from build123d import *

# Parameters (mm, degrees)
SKETCH2_W           = 100
SKETCH2_H           = 77
BOSS_EXTRUDE1_DEPTH = 18
SKETCH3_W           = 100
SKETCH3_H           = 24.402527788
CUT_EXTRUDE1_DEPTH  = 3.5


with BuildPart() as part:
    # Sketch2 → Boss-Extrude1 (new body)
    with BuildSketch(Plane.XY.offset(-10)):
        with Locations((45, 33.5)):
            Rectangle(SKETCH2_W, SKETCH2_H)
    extrude(amount=BOSS_EXTRUDE1_DEPTH)

    # Sketch3 → Cut-Extrude1 (cut)
    with BuildSketch(Plane.XY.offset(8)):
        with Locations((45, 59.798736106)):
            Rectangle(SKETCH3_W, SKETCH3_H)
    extrude(amount=-CUT_EXTRUDE1_DEPTH, mode=Mode.SUBTRACT)


solid = part.part
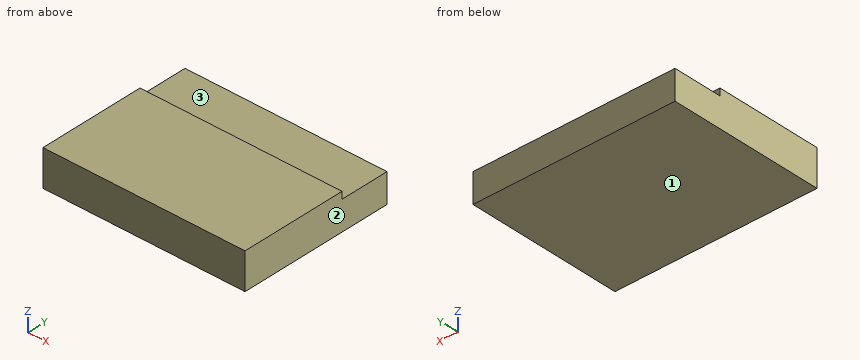
Read the model definition and answer for the solid it produces. Units are mm, in the model's axes. Face numbers are marked on the shaded views. Coordinates: 2 decimals unless noted, no trailing zeros. Loops run counter-clockwise (first coordinate to the right, second up) from the corner with the lowest first, then second, coordinate; pieces in that order, holes last. Notation, with made-up numbers: (18.5, -12.75) -> (54.5, -12.75) arc R22 ccw to (54.5, 16.25) -> close; hole circle Ø3 at (69, 11.25). An arc over 180 degrees is marked (long way). Answer in a Markdown table with one row per item.
Item 1: Straight lines are drawn through the part: line 1 along Y through (x, z) = (50, 7.25); line 2 along Z through (x, y) = (56, 55.5). For each, find the intervals that lie inside material, in ascending order. Write a range as [from, to].
Returned:
| item | result |
|---|---|
| line 1 | y = [-5, 47.6] |
| line 2 | z = [-10, 4.5] |
Item 2: For a pull along Z with two mould halves and no side action, classify the marked faces 1, 2 and 3 as released by +Z, released by -Z, zero draft, split by the parting line, or undercut.
Returned:
| item | result |
|---|---|
| face 1 | released by -Z |
| face 2 | zero draft |
| face 3 | released by +Z |
Item 3: A cutting plane is placed at A-A on x = 50. Determine the outline of the cut face in (y, z), plus the area to 3 significant figures.
Returned:
| item | result |
|---|---|
| outline | (-5, -10) -> (72, -10) -> (72, 4.5) -> (47.6, 4.5) -> (47.6, 8) -> (-5, 8) -> close |
| area | 1,300 mm^2 |
Item 4: Each of these flat-tipped pins is pushed along its axis until it touches: P1, Ø1.8, axis at x = 47.5, z = 5.5, coming from the +Y side; P2, Ø12, axis at x = 60.5, y = 56.5, coming from the +Z side. Where does it stop, or does it pass through?
Returned:
| item | result |
|---|---|
| P1 | stops at y = 47.6 |
| P2 | stops at z = 4.5 |
Item 5: A cutting plane is placed at B-B on y = 50.5. Determine the outline of the cut face in (x, z).
Returned:
| item | result |
|---|---|
| outline | (-5, -10) -> (95, -10) -> (95, 4.5) -> (-5, 4.5) -> close |
